```python
from build123d import *

# Parameters (mm, degrees)
SKETCH1_R           = 4
BOSS_EXTRUDE1_DEPTH = 19.83582727
SKETCH3_R           = 1
CUT_EXTRUDE1_DEPTH  = 22.759137012
SKETCH4_R           = 2.475
CUT_EXTRUDE2_DEPTH  = 2.58519454
BOSS_EXTRUDE2_START = 3
SKETCH5_R           = 6.5
SKETCH5_R_2         = 4
BOSS_EXTRUDE2_DEPTH = 3


with BuildPart() as part:
    # Sketch1 → Boss-Extrude1 (new body)
    with BuildSketch(Plane.XY):
        Circle(SKETCH1_R)
    extrude(amount=BOSS_EXTRUDE1_DEPTH)

    # Sketch3 → Cut-Extrude1 (cut, through all)
    with BuildSketch(Plane(origin=(0, -4, 0), x_dir=(-1, 0, 0), z_dir=(0, -1, 0))):
        with Locations(Location((0, -4.5, 0), (0, 0, 90))):
            Circle(SKETCH3_R)
    extrude(amount=-CUT_EXTRUDE1_DEPTH, mode=Mode.SUBTRACT)

    # Sketch4 → Cut-Extrude2 (cut)
    with BuildSketch(Plane(origin=(0, -4, 0), x_dir=(-1, 0, 0), z_dir=(0, -1, 0))):
        with Locations(Location((0, -4.5, 0), (0, 0, 90))):
            Circle(SKETCH4_R)
    extrude(amount=-CUT_EXTRUDE2_DEPTH, mode=Mode.SUBTRACT)

    # Sketch5 → Boss-Extrude2 (add)
    with BuildSketch(Plane(origin=(0, 0, 12.8359246), x_dir=(-1, 0, 0), z_dir=(0, 0, -1)).offset(BOSS_EXTRUDE2_START)):
        Circle(SKETCH5_R)
        Circle(SKETCH5_R_2, mode=Mode.SUBTRACT)
    extrude(amount=-BOSS_EXTRUDE2_DEPTH)


solid = part.part
```
The model under review builds one solid part; all positions refer to its coordinate system, in mm. A direction names the side the tool comes from. Round coordinates to 2 decimals unless told otherwise and drop trailing zeros. Loops run counter-clockwise (first coordinate to the right, second up) from the corner with the lowest first, then second, coordinate; pieces in that order, holes last.
Item 1: Mouldability with a two-part tool opening along Z and no side actions: class faces 4 (the face through (0, 0, 19.836)), 5 (the face through (0, -1.415, 3)), 6 (the face through (0.74, -2.44, 2.14)), 7 (the face through (-3, 3, 9.836)) as released by +Z, released by -Z, zero draft, split by the parting line, or undercut.
Determined:
face 4: released by +Z
face 5: undercut
face 6: undercut
face 7: released by -Z
Item 2: Take a section at C-C (z = 4.5). Write out the cut boundary in (x, y) (3 decimals).
Determined:
outline: (-2.475, -3.142) - (-2.475, -1.415) - (-1, -1.415) - (-1, 3.873) arc R4 ccw to start; (1, -1.415) - (2.475, -1.415) - (2.475, -3.142) arc R4 ccw to (1, 3.873) - close
Item 3: Take a section at D-D (x = 3.5). Write out the cut boundary in (y, z).
Determined:
outline: (-5.48, 9.84) - (-1.94, 9.84) - (-1.94, 0) - (1.94, 0) - (1.94, 9.84) - (5.48, 9.84) - (5.48, 12.84) - (1.94, 12.84) - (1.94, 19.84) - (-1.94, 19.84) - (-1.94, 12.84) - (-5.48, 12.84) - close
Item 4: Take a section at A-A (x = 0). Write out the cut boundary in (y, z) (3 decimals).
Determined:
outline: (-6.5, 9.836) - (-4, 9.836) - (-4, 6.975) - (-1.415, 6.975) - (-1.415, 5.5) - (4, 5.5) - (4, 9.836) - (6.5, 9.836) - (6.5, 12.836) - (4, 12.836) - (4, 19.836) - (-4, 19.836) - (-4, 12.836) - (-6.5, 12.836) - close; (-4, 0) - (4, 0) - (4, 3.5) - (-1.415, 3.5) - (-1.415, 2.025) - (-4, 2.025) - close
Item 5: For line 1 (Z direction, x = 0, y = -1); line 2 (Z direction, x = 0, y = -2.2) (3 decimals); line 3 (X direction, y = -2.75, z = 6), list the stretches that pass through material, from the lowest coordinate up.
Determined:
line 1: z = 0 to 3.5, 5.5 to 19.84
line 2: z = 0 to 2.025, 6.975 to 19.836
line 3: x = -2.9 to -1.97, 1.97 to 2.9
Item 6: Take a section at B-B (y = 0). Write out the cut boundary in (x, z).
Determined:
outline: (-6.5, 9.84) - (-4, 9.84) - (-4, 0) - (4, 0) - (4, 9.84) - (6.5, 9.84) - (6.5, 12.84) - (4, 12.84) - (4, 19.84) - (-4, 19.84) - (-4, 12.84) - (-6.5, 12.84) - close; hole circle Ø2 at (0, 4.5)
Item 7: Clearance check with flat-ended pins moving along their axes: pin 1 Ø6 at (y, z) = (-1, 2.5) entering from -X; pin 2 Ø4 at (x, z) = (1, 3.5) entering from -Y; pin 3 Ø1.8 at (x, z) = (0, 4.5) entering from -Y; pin 4 Ø4 at (x, y) = (2, -3.5) entering from +Z. State where each tip first meets the part, or that it passes through.
Determined:
pin 1: stops at x = -4
pin 2: stops at y = -4
pin 3: passes through
pin 4: stops at z = 19.84
Item 8: For faces 1 (the face through (-0.6, 1.3, 5.3)), 2 (the face through (-3, 3, 12.836)), 3 (the face through (2.15, 3.373, 4.849)), list the 3-axis set-ups (+Z, -Z, +X, -X, +Y, -Y) from which the entire face can be reached by the end or side of a thin tool; tool diameter is ignored.
Determined:
face 1: +Y, -Y
face 2: +Z
face 3: -Z
